Check sheet for the modelled part. Datum: model origin and axes. Units: mm. Give positions to 0.01 mm unless a question says otherwise; leave off trailing zeros. Loops run counter-clockwise (first coordinate to the right, second up) from the corner with the lowest first, then second, coordinate; pieces in that order, holes last. Notation, with made-up numbers: (37.5, -6) -> (67.5, -6) arc R23 ccw to (67.5, 3) -> close; hole circle Ø1 at (54, -4.75). An arc over 180 degrees is marked (long way). Write each question's results on one line, items separated by ' | '. Start each with the question number.
Item 1: Cross-section at D-D on z = 1.1. State how many separate pieces and enclosed holes the cut face has, then the cut area to 3 significant figures.
Item 2: Cross-section at A-A on y = -61. Enter the section's corners in (x, z), then the cut area to 3 significant figures.
Item 3: Gauge pin test, flat ends, axial feed: pin 1 Ø0.6 at (x, z) = (38.5, 1) entering from +Y; pin 2 Ø1 at (y, z) = (-64, 0.5) entering from -X; pin 3 Ø0.6 at (x, z) = (-39, 1.5) entering from -Y. Record the tip position at first contact, or that the pin passes through.
Item 4: Scan lines: line 1 along X through (y, z) = (-8.5, 1.25); line 2 along X through (y, z) = (46.5, 0.7); line 3 along Y through (x, z) = (36, 0.65). Record each from-to range of solid material in increasing order.
Item 5: Cross-section at B-B on x = 17. Enter the section's corners in (y, z).
Item 6: Cross-section at C-C on x = -27. Enter the section's corners in (y, z), then the cut area to 3 significant figures.
from build123d import *

# Parameters (mm, degrees)
F0_R     = 2
F0_R_2   = 1.5
F0_W     = 2
F0_H     = 5.0564210489
F0_H_2   = 4.9435789511
F1_DEPTH = 2


with BuildPart() as f1:
    # F0 (on Top) → F1 (new body)
    with BuildSketch(Plane.XY):
        Polygon((37.5, 79.9508376047), (-37.5, 79.9508376047), (-37.5, 20), (-37.5, 14.9435789511), (-37.5, 7.5), (-37.5, 0), (-37.5, -7.5), (-37.5, -15.0564210489), (-37.5, -20), (-37.5, -80.0491623953), (37.5, -80.0491623953), (37.5, -20), (37.5, -15.0564210489), (37.5, -7.5), (37.5, 0), (37.5, 7.5), (37.5, 14.9435789511), (37.5, 20), align=None)
        with Locations((-34.5, -76.9508376047)):
            Circle(F0_R, mode=Mode.SUBTRACT)
        Polygon((-32.7663309872, -54.8594370484), (-7.7663309872, -54.8594370484), (-7.7663309872, -74.8594370484), align=None, mode=Mode.SUBTRACT)
        Polygon((-32.7663309872, -49.3169614673), (-32.7663309872, -29.3169614673), (-7.7663309872, -49.3169614673), align=None, mode=Mode.SUBTRACT)
        Polygon((-32.7663309872, -20.8594370484), (-7.7663309872, -20.8594370484), (-7.7663309872, -40.8594370484), align=None, mode=Mode.SUBTRACT)
        Polygon((7.2336690128, -74.8594370484), (7.2336690128, -54.8594370484), (32.2336690128, -54.8594370484), align=None, mode=Mode.SUBTRACT)
        with Locations((34.5, -76.9508376047)):
            Circle(F0_R, mode=Mode.SUBTRACT)
        Polygon((32.2336690128, -49.3169614673), (7.2336690128, -49.3169614673), (32.2336690128, -29.3169614673), align=None, mode=Mode.SUBTRACT)
        Polygon((7.2336690128, -40.8594370484), (7.2336690128, -20.8594370484), (32.2336690128, -20.8594370484), align=None, mode=Mode.SUBTRACT)
        with BuildLine():
            ThreePointArc((-34.5, 0), (-36, -1.5), (-37.5, 0))
            ThreePointArc((-37.5, 0), (-36, 1.5), (-34.5, 0))
        make_face(mode=Mode.SUBTRACT)
        Polygon((-7.7663309872, 41.1405629516), (-7.7663309872, 21.1405629516), (-32.7663309872, 21.1405629516), align=None, mode=Mode.SUBTRACT)
        Polygon((-7.7663309872, 49.5980873704), (-32.7663309872, 29.5980873704), (-32.7663309872, 49.5980873704), align=None, mode=Mode.SUBTRACT)
        with Locations((-34.5, 76.9508376047)):
            Circle(F0_R, mode=Mode.SUBTRACT)
        Polygon((-7.7663309872, 55.1405629516), (-32.7663309872, 55.1405629516), (-7.7663309872, 75.1405629516), align=None, mode=Mode.SUBTRACT)
        Polygon((32.2336690128, 21.1405629516), (7.2336690128, 21.1405629516), (7.2336690128, 41.1405629516), align=None, mode=Mode.SUBTRACT)
        Polygon((32.2336690128, 49.5980873704), (32.2336690128, 29.5980873704), (7.2336690128, 49.5980873704), align=None, mode=Mode.SUBTRACT)
        with Locations((36, 0)):
            Circle(F0_R_2, mode=Mode.SUBTRACT)
        Polygon((32.2336690128, 55.1405629516), (7.2336690128, 55.1405629516), (7.2336690128, 75.1405629516), align=None, mode=Mode.SUBTRACT)
        with Locations((34.5, 76.9508376047)):
            Circle(F0_R, mode=Mode.SUBTRACT)
        Polygon((39.5, 7.5), (37.5, 7.5), (37.5, 0), (37.5, -7.5), (39.5, -7.5), (39.5, -5), (39.5, 5), align=None)
        Polygon((-37.5, 0), (-37.5, 7.5), (-39.5, 7.5), (-39.5, 5), (-39.5, -5), (-39.5, -7.5), (-37.5, -7.5), align=None)
        with Locations((38.5, 17.4717894755)):
            Rectangle(F0_W, F0_H)
        with Locations((38.5, -17.5282105245)):
            Rectangle(F0_W, F0_H_2)
        with Locations((-38.5, -17.5282105245)):
            Rectangle(F0_W, F0_H_2)
        with Locations((-38.5, 17.4717894755)):
            Rectangle(F0_W, F0_H)
        Polygon((-39.5, 14.9435789511), (-39.5, 20), (-42.5, 20), (-42.5, 5), (-39.5, 5), (-39.5, 7.5), align=None)
        Polygon((42.5, 20), (39.5, 20), (39.5, 14.9435789511), (39.5, 7.5), (39.5, 5), (42.5, 5), align=None)
        Polygon((42.5, -20), (42.5, -5), (39.5, -5), (39.5, -7.5), (39.5, -15.0564210489), (39.5, -20), align=None)
        Polygon((-39.5, -5), (-42.5, -5), (-42.5, -20), (-39.5, -20), (-39.5, -15.0564210489), (-39.5, -7.5), align=None)
    extrude(amount=F1_DEPTH)


solid = f1.part
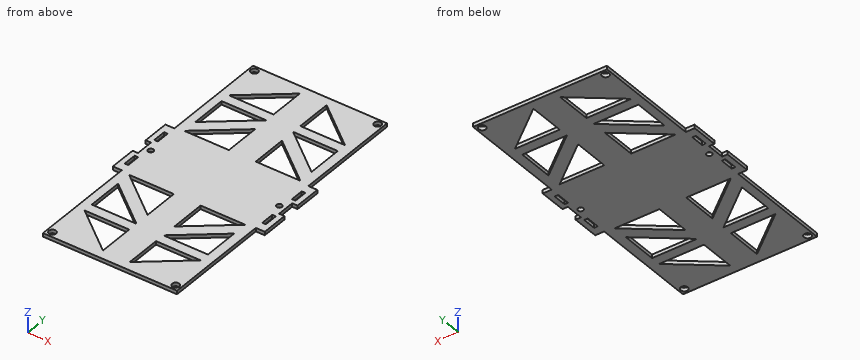
Answer sheet:
1) separate pieces: 1 | enclosed holes: 22 | area: 9,220 mm²
2) outline: (-37.5, 0) -> (-25.09, 0) -> (-25.09, 2) -> (-37.5, 2) -> close; (-7.77, 0) -> (7.23, 0) -> (7.23, 2) -> (-7.77, 2) -> close; (24.56, 0) -> (37.5, 0) -> (37.5, 2) -> (24.56, 2) -> close | area: 80.7 mm²
3) pin 1: stops at y = 20 | pin 2: stops at x = -37.5 | pin 3: stops at y = -20
4) line 1: x = -42.5 to -39.5, -37.5 to 37.5, 39.5 to 42.5 | line 2: x = -37.5 to -32.77, -11.64 to 11.11, 32.23 to 37.5 | line 3: y = -80.05 to -78.27, -75.63 to -1.5, 1.5 to 75.63, 78.27 to 79.95
5) outline: (-80.05, 0) -> (-67.05, 0) -> (-67.05, 2) -> (-80.05, 2) -> close; (-54.86, 0) -> (-49.32, 0) -> (-49.32, 2) -> (-54.86, 2) -> close; (-41.5, 0) -> (-33.05, 0) -> (-33.05, 2) -> (-41.5, 2) -> close; (-20.86, 0) -> (21.14, 0) -> (21.14, 2) -> (-20.86, 2) -> close; (33.33, 0) -> (41.79, 0) -> (41.79, 2) -> (33.33, 2) -> close; (49.6, 0) -> (55.14, 0) -> (55.14, 2) -> (49.6, 2) -> close; (67.33, 0) -> (79.95, 0) -> (79.95, 2) -> (67.33, 2) -> close
6) outline: (-80.05, 0) -> (-59.47, 0) -> (-59.47, 2) -> (-80.05, 2) -> close; (-54.86, 0) -> (-49.32, 0) -> (-49.32, 2) -> (-54.86, 2) -> close; (-33.93, 0) -> (-25.47, 0) -> (-25.47, 2) -> (-33.93, 2) -> close; (-20.86, 0) -> (21.14, 0) -> (21.14, 2) -> (-20.86, 2) -> close; (25.75, 0) -> (34.21, 0) -> (34.21, 2) -> (25.75, 2) -> close; (49.6, 0) -> (55.14, 0) -> (55.14, 2) -> (49.6, 2) -> close; (59.75, 0) -> (79.95, 0) -> (79.95, 2) -> (59.75, 2) -> close | area: 222 mm²
